For this review, take the finished solid that the model builds, in its own axes (mm). A direction names the side the tool comes from. Round coordinates to 2 decimals unless told otherwise and drop trailing zeros. Loops run counter-clockwise (first coordinate to the right, second up) from the corner with the lowest first, then second, coordinate; pieces in that order, holes last.
1) Take a section at B-B (y = -0.95). State the section outline as (x, z) points.
2) Tool access review of faces 1 (the flat face through (7, 0, 18.3)), 2 (the flat face through (-4.25, 0, 9)): name each direction out of +Z, -Z, +X, -X, +Y, -Y from which nothing blocks a thin tool from reaching the whole face with its end or side.
3) Insertion check: pin 1 (0.9 mm diameter, centred on y = -0.5, z = 27, fed in from -X); pin 2 (8 mm diameter, centred on x = 5.5, z = 22.5, fed in from +Y). Each pin has a flat end and moves straight along its axis. Give the tip position at first contact, or say it passes through.
4) Wall thickness on L1, parallel to Z at x = 10, y = 0.1; L2, parallel to X at y = -0.05, z = 26; L3, parallel to X at y = 1.15, z = 11: over which ranges is each line inside the solid? List them lowest first.
5) Take a section at C-C (x = 12). State the section outline as (y, z) points, then the cut area to 3 significant figures.
```python
from build123d import *

# Parameters (mm, degrees)
SKETCH1_W           = 53.5
SKETCH1_H           = 3
BOSS_EXTRUDE1_DEPTH = 30.3
SKETCH2_W           = 23.75
SKETCH2_H           = 3
CUT_EXTRUDE1_DEPTH  = 12
FILLET1_R           = 1.5


with BuildPart() as part:
    # Sketch1 → Boss-Extrude1 (new body)
    with BuildSketch(Plane.XY):
        with Locations((22.5, 0)):
            Rectangle(SKETCH1_W, SKETCH1_H)
    extrude(amount=BOSS_EXTRUDE1_DEPTH)

    # Sketch2 → Cut-Extrude1 (cut)
    with BuildSketch(Plane.XY.offset(30.3)):
        with Locations((7.625, 0)):
            Rectangle(SKETCH2_W, SKETCH2_H)
    extrude(amount=-CUT_EXTRUDE1_DEPTH, mode=Mode.SUBTRACT)

    # Fillet1
    fillet1_edges = [part.edges().sort_by_distance(p)[0] for p in [
        (49.25, -1.5, 15.15),
        (49.25, 1.5, 15.15),
    ]]
    fillet(fillet1_edges, radius=FILLET1_R - 0.0001)  # a hair under: the kernel refuses the full size


solid = part.part
```
Response:
1. outline: (-4.25, 0) - (48.91, 0) - (48.91, 30.3) - (19.5, 30.3) - (19.5, 18.3) - (-4.25, 18.3) - close
2. face 1: +Z, -X, +Y, -Y
2. face 2: +Z, -Z, -X, +Y, -Y
3. pin 1: stops at x = 19.5
3. pin 2: passes through
4. L1: z = 0 to 18.3
4. L2: x = 19.5 to 49.25
4. L3: x = -4.25 to 48.71
5. outline: (-1.5, 0) - (1.5, 0) - (1.5, 18.3) - (-1.5, 18.3) - close
5. area: 54.9 mm2
